Geometry: final body of the model. Coordinates: model frame, mm. A direction names the side the tool comes from. Give positions to 0.01 mm unless a question says otherwise; leave off trailing zeros. Order: outer loops, then holes, each group sorted by start corner. A loop starts at its lowest first (then second) coordinate and runs counter-clockwise, first axis right, second up. Notation, with made-up numbers: (7, 22.25) - (59, 22.25) arc R31 cw to (59, 47.25) - close; hole circle Ø8 at (2.25, 31). An arc over 180 degrees is marked (long way). Use one line per item in the form item = value.
from build123d import *

# Parameters (mm, degrees)
BOSS_EXTRUDE1_DEPTH       = 17.78
CUT_EXTRUDE1_DEPTH        = 16.78
CUT_EXTRUDE1_DEPTH_BACK   = 16.78
SKETCH4_R                 = 8
CUT_EXTRUDE2_DEPTH        = 91.122241428
SKETCH5_R                 = 11.2
CUT_EXTRUDE3_DEPTH        = 96.309067774
BOSS_EXTRUDE2_DEPTH       = 2
M3X0_5_TAPPED_HOLE2_D     = 2.5
M3X0_5_TAPPED_HOLE2_DEPTH = 7.5
M3X0_5_TAPPED_HOLE2_TIP   = 0.751075774
FILLET6_R                 = 2
M3_CLEARANCE_HOLE1_D      = 3.4
M3_CLEARANCE_HOLE1_DEPTH  = 12.7


with BuildPart() as part:
    # Sketch1 → Boss-Extrude1 (new, symmetric)
    with BuildSketch(Plane.XY):
        Polygon((0, -15), (0, 15), (0, 17), (2, 17), (88.7, 17), (88.7, 15), (2, -15), align=None)
    extrude(amount=BOSS_EXTRUDE1_DEPTH, both=True)

    # Sketch2 → Cut-Extrude1 (cut, two sides: drawn at the far end of the back side and taken through both)
    with BuildSketch(Plane.XY.offset(-CUT_EXTRUDE1_DEPTH_BACK)):
        Polygon((2, 15), (2, -15), (88.7, 15), align=None)
    extrude(amount=CUT_EXTRUDE1_DEPTH + CUT_EXTRUDE1_DEPTH_BACK, mode=Mode.SUBTRACT)

    # Sketch4 → Cut-Extrude2 (cut, through all)
    with BuildSketch(Plane(origin=(2, 0, 0), x_dir=(0, 0, -1), z_dir=(1, 0, 0))):
        with Locations(Location((0, -1, 0), (0, 0, 90))):
            Circle(SKETCH4_R)
    extrude(amount=-CUT_EXTRUDE2_DEPTH, mode=Mode.SUBTRACT)

    # Sketch5 → Cut-Extrude3 (cut, through all)
    with BuildSketch(Plane.XZ.offset(-15)):
        with Locations((65, 0)):
            Circle(SKETCH5_R)
    extrude(amount=-CUT_EXTRUDE3_DEPTH, mode=Mode.SUBTRACT)

    # Sketch7 → Boss-Extrude2 (add)
    with BuildSketch(Plane.XZ.offset(-15)):
        with BuildLine():
            Line((49.484209973, -12.515790027), (49.484209973, -16.78))
            Line((49.484209973, -16.78), (55.484209973, -16.78))
            Line((55.484209973, -16.78), (55.484209973, -12.515790027))
            ThreePointArc((55.484209973, -12.515790027), (52.484209973, -9.515790027), (49.484209973, -12.515790027))
        make_face()
        with BuildLine():
            Line((74.515790027, -12.515790027), (74.515790027, -16.78))
            Line((74.515790027, -16.78), (80.515790027, -16.78))
            Line((80.515790027, -16.78), (80.515790027, -12.515790027))
            ThreePointArc((80.515790027, -12.515790027), (77.515790027, -9.515790027), (74.515790027, -12.515790027))
        make_face()
        with BuildLine():
            Line((80.515790027, 12.515790027), (80.515790027, 16.78))
            Line((80.515790027, 16.78), (74.515790027, 16.78))
            Line((74.515790027, 16.78), (74.515790027, 12.515790027))
            ThreePointArc((74.515790027, 12.515790027), (77.515790027, 9.515790027), (80.515790027, 12.515790027))
        make_face()
        with BuildLine():
            Line((49.484209973, 12.515790027), (49.484209973, 16.78))
            Line((49.484209973, 16.78), (55.484209973, 16.78))
            Line((55.484209973, 16.78), (55.484209973, 12.515790027))
            ThreePointArc((55.484209973, 12.515790027), (52.484209973, 9.515790027), (49.484209973, 12.515790027))
        make_face()
    extrude(amount=BOSS_EXTRUDE2_DEPTH)

    # M3x0.5 Tapped Hole2
    with Locations(Plane(origin=(0, 13, 0), x_dir=(-1, 0, 0), z_dir=(0, -1, 0))):
        with Locations((-52.484209973, -12.515790027), (-77.515790027, -12.515790027), (-77.515790027, 12.515790027), (-52.484209973, 12.515790027)):
            Hole(M3X0_5_TAPPED_HOLE2_D / 2, depth=M3X0_5_TAPPED_HOLE2_DEPTH)
            with Locations((0, 0, -(M3X0_5_TAPPED_HOLE2_DEPTH + M3X0_5_TAPPED_HOLE2_TIP / 2))):  # 118° drill point
                Cone(0, M3X0_5_TAPPED_HOLE2_D / 2, M3X0_5_TAPPED_HOLE2_TIP, mode=Mode.SUBTRACT)

    # Fillet6
    fillet6_edges = [part.edges().sort_by_distance(p)[0] for p in [
        (2, 0, -16.78),
        (2, 0, 16.78),
        (49.484209973, 14, -16.78),
        (55.484209973, 14, -16.78),
        (74.515790027, 14, -16.78),
        (80.515790027, 14, -16.78),
        (80.515790027, 14, 16.78),
        (74.515790027, 14, 16.78),
        (55.484209973, 14, 16.78),
        (49.484209973, 14, 16.78),
    ]]
    fillet(fillet6_edges, radius=FILLET6_R)

    # M3 Clearance Hole1
    with Locations(Plane.ZY):
        with Locations((0, 9), (10, -1), (0, -11), (-10, -1)):
            Hole(M3_CLEARANCE_HOLE1_D / 2, depth=M3_CLEARANCE_HOLE1_DEPTH)


solid = part.part
(1) Cut plane A-A on y = -1. Output: boundary loops of the cut face in (x, z), plus the area to 3 significant figures.
Computed values:
outline = (0, -17.78) - (42.46, -17.78) - (42.46, -16.78) - (4, -16.78) arc R2 cw to (2, -14.78) - (2, -11.7) - (0, -11.7) - close; (0, -8.3) - (2, -8.3) - (2, -8) - (0, -8) - close; (0, 8) - (2, 8) - (2, 8.3) - (0, 8.3) - close; (0, 11.7) - (2, 11.7) - (2, 14.78) arc R2 cw to (4, 16.78) - (42.46, 16.78) - (42.46, 17.78) - (0, 17.78) - close
area = 108 mm²
(2) Reachability of faces 4 (the face through (80.516, 14, 14)), 5 (the face through (45.55, 0.07, 17.4)), 6 (the face through (49.484, 14, 14)) from +Z, -Z, +X, -X, +Y, -Y: full face, straight path, thin tool, end or side. Return the list, or none.
Computed values:
face_4 = +X, -Y
face_5 = +Z, -Z, +X, -Y
face_6 = -Y
(3) Cut plane C-C on y = -11. Output: boundary loops of the cut face in (x, z), plus the area to 3 significant figures.
Computed values:
outline = (0, -17.78) - (13.56, -17.78) - (13.56, -16.78) - (4, -16.78) arc R2 cw to (2, -14.78) - (2, -1.7) - (0, -1.7) - close; (0, 1.7) - (2, 1.7) - (2, 14.78) arc R2 cw to (4, 16.78) - (13.56, 16.78) - (13.56, 17.78) - (0, 17.78) - close
area = 89.2 mm²
(4) Contact query for flat-ended pins moving along their axis: pin 1 Ø1 at (y, z) = (14, -13) entering from +X; pin 2 Ø3 at (y, z) = (-1, -10) entering from +X; pin 3 Ø10 at (y, z) = (-7.5, -7.5) entering from +X; pin 4 Ø3 at (x, z) = (52.48, 12.52) entering from -Y. Output: stop coordinate, or through.
Computed values:
pin_1 = 80.52
pin_2 = through
pin_3 = 2
pin_4 = 13
(5) Ray query, line 1 along Z through (x, y) = (15.5, 7); line 2 along X through (y, z) = (6, 14.5); line 3 along Y through (x, z) = (39, -10.5). Return the intervals inside material, ascending.
Computed values:
line_1 = -17.78 to -16.78, 16.78 to 17.78
line_2 = 0 to 2
line_3 = 15 to 17
(6) Cut plane D-D on z = 6. Output: boundary loops of the cut face in (x, y), plus the area to 3 significant figures.
Computed values:
outline = (0, -15) - (2, -15) - (2, -6.29) - (0, -6.29) - close; (0, 4.29) - (2, 4.29) - (2, 15) - (55.54, 15) - (55.54, 17) - (0, 17) - close; (74.46, 15) - (88.7, 15) - (88.7, 17) - (74.46, 17) - close
area = 178 mm²
(7) Cut plane B-B on z = 0. Output: boundary loops of the cut face in (x, y), plus the area to 3 significant figures.
Computed values:
outline = (0, -15) - (2, -15) - (2, -12.7) - (0, -12.7) - close; (0, -9.3) - (2, -9.3) - (2, -9) - (0, -9) - close; (0, 7) - (2, 7) - (2, 7.3) - (0, 7.3) - close; (0, 10.7) - (2, 10.7) - (2, 15) - (53.8, 15) - (53.8, 17) - (0, 17) - close; (76.2, 15) - (88.7, 15) - (88.7, 17) - (76.2, 17) - close
area = 147 mm²
(8) Pull-direction query (Y, two-part tool) for faces 1 (the face through (1.01, 7.34, 0.37)), 2 (the face through (81.12, 13.99, 16.21)), 3 (the face through (1, -15, 0)); classes: released by +Y, released by -Y, zero draft, split by the parting line, or undercut.
Computed values:
face_1 = undercut
face_2 = zero draft
face_3 = released by -Y
